Verification items for the finished model (mm, model axes). A direction names the side the tool comes from. Coordinates: 2 decimals unless noted, no trailing zeros. Loops run counter-clockwise (first coordinate to the right, second up) from the corner with the lowest first, then second, coordinate; pieces in that order, holes last. Notation, with made-up numbers: (26, -39) -> (31, -39) arc R16 ccw to (31, -24) -> close; hole circle Ø8 at (-21, 37.5). An arc over 180 degrees is marked (long way). Answer as a JSON object with one key per item and string values. Group by question number.
Q1. Cross-section at D-D on z = -21. Record the boundary of the cut face in (x, y), and give its area (3 significant figures).
Q2. Cross-section at B-B on x = 0. Record the boundary of the cut face in (y, z), and give its area (4 significant figures).
Q3. Scan lines: L1, parallel to Y at x = 0, z = 32; L2, parallel to Z at x = 0, y = -10.5; L3, parallel to Z at x = 3, y = 8.5. Record each from-to range of solid material in increasing order.
Q4. Gauge pin test, flat ends, axial feed: pin 1 Ø4 at (y, z) = (-15, 33) entering from -X; pin 2 Ø8 at (x, z) = (6.5, -14) entering from -Y; pin 3 Ø3 at (y, z) = (-6, -8.5) entering from +X. Record the tip position at first contact, or that the pin passes through.
Q5. Set-up check for faces 1 (the flat face through (13, 0, 28.5)), 2 (the flat face through (0, 2.5, 47)), 3 (the cylindrical face through (-8.767, -16.856, -29.58)): record each of +Z, -Z, +X, -X, +Y, -Y from which the full face is reachable in a straight line by a thin tool's end or side.
Q6. Cross-section at C-C on y = 0. Record the boundary of the cut face in (x, z), and give its area (3 significant figures).
Q7. Release check for a two-part mould opening along Y. For faces 4 (the flat face through (0, 0, 53)), 5 (the cylindrical face through (-0.65, -2.93, 44.63)), 6 (the cylindrical face through (-14.5, 0.07, 31.04)) record: released by +Y, released by -Y, zero draft, split by the parting line, or undercut.
Q8. Cross-section at A-A on z = 30. Record the boundary of the cut face in (x, y), and give its area (3 significant figures).
```python
from build123d import *

# Parameters (mm, degrees)
SKETCH_1_R          = 16
EXTRUDE_1_DEPTH     = 33.5
SKETCH_2_R          = 10
EXTRUDE_2_DEPTH     = 3
SKETCH_3_R          = 3
EXTRUDE_3_DEPTH     = 16.5
CUT_EXTRUDE_START   = 3
SKETCH_4_W          = 9.243576196
SKETCH_4_H          = 12
CUT_EXTRUDE_1_DEPTH = 0.5
SKETCH_5_R          = 19
EXTRUDE_4_DEPTH     = 60
SKETCH_6_R          = 1.5
CUT_EXTRUDE_2_DEPTH = 5


with BuildPart() as part:
    # ｽｹｯﾁ1 → ﾎﾞｽ - 押し出し1 (new body)
    with BuildSketch(Plane.XY):
        Circle(SKETCH_1_R)
    extrude(amount=EXTRUDE_1_DEPTH)

    # ｽｹｯﾁ2 → ﾎﾞｽ - 押し出し2 (add)
    with BuildSketch(Plane.XY.offset(33.5)):
        Circle(SKETCH_2_R)
    extrude(amount=EXTRUDE_2_DEPTH)

    # ｽｹｯﾁ3 → ﾎﾞｽ - 押し出し3 (add)
    with BuildSketch(Plane.XY.offset(36.5)):
        Circle(SKETCH_3_R)
    extrude(amount=EXTRUDE_3_DEPTH)

    # ｽｹｯﾁ4 → ｶｯﾄ - 押し出し1 (cut)
    with BuildSketch(Plane(origin=(0, 0, 0), x_dir=(1, 0, 0), z_dir=(0, 1, 0)).offset(CUT_EXTRUDE_START)):
        with Locations((0, -47)):
            Rectangle(SKETCH_4_W, SKETCH_4_H)
    extrude(amount=-CUT_EXTRUDE_1_DEPTH, mode=Mode.SUBTRACT)

    # ｽｹｯﾁ5 → ﾎﾞｽ - 押し出し4 (add)
    with BuildSketch(Plane(origin=(0, 0, 0), x_dir=(-1, 0, 0), z_dir=(0, 0, -1))):
        Circle(SKETCH_5_R)
    extrude(amount=EXTRUDE_4_DEPTH)

    # ｽｹｯﾁ6 → ｶｯﾄ - 押し出し2 (cut)
    with BuildSketch(Plane.XY.offset(33.5)):
        with Locations((0, 13)):
            Circle(SKETCH_6_R)
        with Locations((-13, 0)):
            Circle(SKETCH_6_R)
        with Locations(Location((13, 0, 0), (0, 0, 180))):
            Circle(SKETCH_6_R)
        with Locations(Location((0, -13, 0), (0, 0, 180))):
            Circle(SKETCH_6_R)
    extrude(amount=-CUT_EXTRUDE_2_DEPTH, mode=Mode.SUBTRACT)


solid = part.part
```
Computed values:
{
 "1": {"outline": "circle Ø38 at (0, 0)", "area": "1,130 mm²"},
 "2": {"outline": "(-19, -60) -> (19, -60) -> (19, 0) -> (16, 0) -> (16, 33.5) -> (14.5, 33.5) -> (14.5, 28.5) -> (11.5, 28.5) -> (11.5, 33.5) -> (10, 33.5) -> (10, 36.5) -> (3, 36.5) -> (3, 41) -> (2.5, 41) -> (2.5, 53) -> (-3, 53) -> (-3, 36.5) -> (-10, 36.5) -> (-10, 33.5) -> (-11.5, 33.5) -> (-11.5, 28.5) -> (-14.5, 28.5) -> (-14.5, 33.5) -> (-16, 33.5) -> (-16, 0) -> (-19, 0) -> close", "area": "3,475 mm²"},
 "3": {"L1": "y = -16 to -14.5, -11.5 to 11.5, 14.5 to 16", "L2": "z = -60 to 33.5", "L3": "z = -60 to 36.5"},
 "4": {"pin 1": "stops at x = -9.33", "pin 2": "stops at y = -18.83", "pin 3": "stops at x = 18.46"},
 "5": {"face 1": "+Z", "face 2": "+Z, +X, -X, +Y", "face 3": "+Z, -Z"},
 "6": {"outline": "(-19, -60) -> (19, -60) -> (19, 0) -> (16, 0) -> (16, 33.5) -> (14.5, 33.5) -> (14.5, 28.5) -> (11.5, 28.5) -> (11.5, 33.5) -> (10, 33.5) -> (10, 36.5) -> (3, 36.5) -> (3, 53) -> (-3, 53) -> (-3, 36.5) -> (-10, 36.5) -> (-10, 33.5) -> (-11.5, 33.5) -> (-11.5, 28.5) -> (-14.5, 28.5) -> (-14.5, 33.5) -> (-16, 33.5) -> (-16, 0) -> (-19, 0) -> close", "area": "3,480 mm²"},
 "7": {"face 4": "zero draft", "face 5": "split by the parting line", "face 6": "undercut"},
 "8": {"outline": "circle Ø32 at (0, 0); hole circle Ø3 at (-13, 0); hole circle Ø3 at (0, -13); hole circle Ø3 at (0, 13); hole circle Ø3 at (13, 0)", "area": "776 mm²"}
}
